from build123d import *

# Parameters (mm, degrees)
SKETCH_W        = 15
SKETCH_H        = 23.9
PAD_DEPTH       = 3
SKETCH001_W     = 15
SKETCH001_H     = 7.6
PAD001_DEPTH    = 4
PAD002_DEPTH    = 2.6
SKETCH003_W     = 4.8
SKETCH003_H     = 0.5
POCKET_DEPTH    = 20
SKETCH004_W     = 2.45
SKETCH004_H     = 1.4
POCKET001_DEPTH = 20
SKETCH005_W     = 15
SKETCH005_H     = 2.5
PAD003_DEPTH    = 25


with BuildPart() as part:
    # Sketch → Pad (new body)
    with BuildSketch(Plane.XY):
        Rectangle(SKETCH_W, SKETCH_H)
    extrude(amount=PAD_DEPTH)

    # Sketch001 → Pad001 (new body)
    with BuildSketch(Plane.XY.offset(3)):
        Rectangle(SKETCH001_W, SKETCH001_H)
    extrude(amount=PAD001_DEPTH)

    # Sketch002 → Pad002 (new body)
    with BuildSketch(Plane.XY.offset(3)):
        Polygon((-3.1, -11.95), (3.1, -11.95), (3.1, -5.6), (4.5, -3.8), (-4.5, -3.8), (-3.1, -5.6), align=None)
    extrude(amount=PAD002_DEPTH)

    # Sketch003 → Pocket (cut)
    with BuildSketch(Plane(origin=(0, 0, 0), x_dir=(1, 0, 0), z_dir=(0, 0, -1))):
        with Locations((0, 11.7)):
            Rectangle(SKETCH003_W, SKETCH003_H)
        with Locations((0, -11.7)):
            Rectangle(SKETCH003_W, SKETCH003_H)
    extrude(amount=-POCKET_DEPTH, mode=Mode.SUBTRACT)

    # Sketch004 → Pocket001 (cut)
    with BuildSketch(Plane.YZ.offset(7.5)):
        with Locations((0, 0.7)):
            Rectangle(SKETCH004_W, SKETCH004_H)
    extrude(amount=-POCKET001_DEPTH, mode=Mode.SUBTRACT)

    # Sketch005 → Pad003 (new body)
    with BuildSketch(Plane(origin=(0, 0, 0), x_dir=(1, 0, 0), z_dir=(0, 0, -1))):
        with Locations((0, 8.7)):
            Rectangle(SKETCH005_W, SKETCH005_H)
    extrude(amount=PAD003_DEPTH)


solid = part.part
Can you work these out from the model? Positions are in its coordinate system, mm. A direction names the side the tool comes from. Round coordinates to 2 decimals unless told otherwise and drop trailing zeros. Loops run counter-clockwise (first coordinate to the right, second up) from the corner with the lowest first, then second, coordinate; pieces in that order, holes last. Notation, with made-up numbers: (20.25, 66.5) - (35.25, 66.5) arc R27 cw to (35.25, 105.5) - close; hole circle Ø1 at (75.5, 44.5). An arc over 180 degrees is marked (long way). Answer in a Markdown table with one row per item. Add a question column.
Q1. We'd pull the mould along X, two halves only. Please class faces 6 (the flat face through (0, 11.45, 1)), 7 (the flat face through (3.8, -4.7, 4.3)), 8 (the flat face through (5, -8, 3)): pulls with the +X half, pulls with the -X half, needs draft (parallel to the pull), parting line crosses it, or undercut.
Q2. For pin 1 Ø6.5 at (x, y) = (2, -9.5) entering from +Z; pin 2 Ø0.8 at (y, z) = (-10, 4.5) entering from +X; pin 3 Ø3.5 at (x, y) = (-5.5, -9) entering from +Z, each with a flat end and sliding along its axis, tell me the tip position at first contact or that it passes through.
Q3. I want a section at D-D on x = 5. List the corners of the cut face in (y, z) for me (3 decimals).
Q4. I need wall thicknesses on L1, parallel to Y at x = -5, z = 0.5 (3 decimals); L2, parallel to Y at x = -1.5, z = -1; L3, parallel to Z at x = -3, y = -5.5. Which ranges of each line are inside material? Lowest first, please.
Q5. I want a section at B-B on y = -9. List the corners of the cut face in (x, z) for me.
Q6. Which directions (+Z, -Z, +X, -X, +Y, -Y) give clear straight access to the entire face, cutting with the end or side of a thin tool? Please do faces 1 (the flat face through (0, 1.225, 1)), 2 (the flat face through (0, -8, 5.6)), 3 (the flat face through (0, -4, 0)), 4 (the flat face through (0, -9.95, -12)), 5 (the flat face through (0, 3.8, 5)).
Q7. I want a section at C-C on z = 4. List the corners of the cut face in (x, y) for me, and give its area (3 significant figures).
Q8. I want a section at A-A on x = 0.25. List the corners of the cut face in (y, z) for me (3 decimals), and give its area (3 significant figures).
A:
| question | item | result |
|---|---|---|
| 1 | face 6 | undercut |
| 1 | face 7 | pulls with the +X half |
| 1 | face 8 | needs draft |
| 2 | pin 1 | z = 5.6 |
| 2 | pin 2 | x = 3.1 |
| 2 | pin 3 | z = 3 |
| 3 | outline | (-11.95, 0) - (-9.95, 0) - (-9.95, -25) - (-7.45, -25) - (-7.45, 0) - (-1.225, 0) - (-1.225, 1.4) - (1.225, 1.4) - (1.225, 0) - (11.95, 0) - (11.95, 3) - (3.8, 3) - (3.8, 7) - (-3.8, 7) - (-3.8, 3) - (-11.95, 3) - close |
| 4 | L1 | -11.95 to -1.225, 1.225 to 11.95 |
| 4 | L2 | -9.95 to -7.45 |
| 4 | L3 | 0 to 5.6 |
| 5 | outline | (-7.5, -25) - (7.5, -25) - (7.5, 3) - (3.1, 3) - (3.1, 5.6) - (-3.1, 5.6) - (-3.1, 3) - (-7.5, 3) - close |
| 6 | face 1 | -Z, +X, -X |
| 6 | face 2 | +Z, +X, -X, -Y |
| 6 | face 3 | -Z, +X, -X, +Y |
| 6 | face 4 | -Z, +X, -X, -Y |
| 6 | face 5 | +Z, +X, -X, +Y |
| 7 | outline | (-7.5, -3.8) - (-4.5, -3.8) - (-3.1, -5.6) - (-3.1, -11.95) - (-2.4, -11.95) - (-2.4, -11.45) - (2.4, -11.45) - (2.4, -11.95) - (3.1, -11.95) - (3.1, -5.6) - (4.5, -3.8) - (7.5, -3.8) - (7.5, 3.8) - (-7.5, 3.8) - close |
| 7 | area | 165 mm^2 |
| 8 | outline | (-11.45, 0) - (-9.95, 0) - (-9.95, -25) - (-7.45, -25) - (-7.45, 0) - (-1.225, 0) - (-1.225, 1.4) - (1.225, 1.4) - (1.225, 0) - (11.45, 0) - (11.45, 3) - (3.8, 3) - (3.8, 7) - (-3.8, 7) - (-3.8, 5.6) - (-11.45, 5.6) - close |
| 8 | area | 178 mm^2 |
